from build123d import *

# Parameters (mm, degrees)
SKETCH_1_R      = 60
SKETCH_1_R_2    = 5
EXTRUDE_1_DEPTH = 3
FILLET_1_R      = 2
FILLET_2_R      = 2
FILLET_4_R      = 2


with BuildPart() as part:
    # 草图1 → 凸台-拉伸1 (new body)
    with BuildSketch(Plane.XY):
        Circle(SKETCH_1_R)
        Circle(SKETCH_1_R_2, mode=Mode.SUBTRACT)
        with BuildLine():
            Line((3, 54.918120871), (3, 9.539392014))
            ThreePointArc((3, 9.539392014), (7.071067812, 7.071067812), (9.539392014, 3))
            Line((9.539392014, 3), (54.918120871, 3))
            ThreePointArc((54.918120871, 3), (38.890872965, 38.890872965), (3, 54.918120871))
        make_face(mode=Mode.SUBTRACT)
        with BuildLine():
            Line((-9.539392014, -3), (-54.918120871, -3))
            ThreePointArc((-54.918120871, -3), (-38.890872965, -38.890872965), (-3, -54.918120871))
            Line((-3, -54.918120871), (-3, -9.539392014))
            ThreePointArc((-3, -9.539392014), (-7.071067812, -7.071067812), (-9.539392014, -3))
        make_face(mode=Mode.SUBTRACT)
        with BuildLine():
            Line((9.539392014, -3), (54.918120871, -3))
            ThreePointArc((54.918120871, -3), (38.890872965, -38.890872965), (3, -54.918120871))
            Line((3, -54.918120871), (3, -9.539392014))
            ThreePointArc((3, -9.539392014), (7.071067812, -7.071067812), (9.539392014, -3))
        make_face(mode=Mode.SUBTRACT)
        with BuildLine():
            Line((-3, 9.539392014), (-3, 54.918120871))
            ThreePointArc((-3, 54.918120871), (-38.890872965, 38.890872965), (-54.918120871, 3))
            Line((-54.918120871, 3), (-9.539392014, 3))
            ThreePointArc((-9.539392014, 3), (-7.071067812, 7.071067812), (-3, 9.539392014))
        make_face(mode=Mode.SUBTRACT)
    extrude(amount=EXTRUDE_1_DEPTH)

    # 圆角1
    fillet_1_edges = [part.edges().sort_by_distance(p)[0] for p in [
        (3, 54.918120871, 1.5),
    ]]
    fillet(fillet_1_edges, radius=FILLET_1_R)

    # 圆角2
    fillet_2_edges = [part.edges().sort_by_distance(p)[0] for p in [
        (54.918120871, 3, 1.5),
        (3, -54.918120871, 1.5),
        (54.918120871, -3, 1.5),
        (-54.918120871, -3, 1.5),
        (-3, -54.918120871, 1.5),
        (-3, 54.918120871, 1.5),
        (-54.918120871, 3, 1.5),
    ]]
    fillet(fillet_2_edges, radius=FILLET_2_R)

    # 圆角4
    fillet_4_edges = [part.edges().sort_by_distance(p)[0] for p in [
        (3, 9.539392014, 1.5),
        (9.539392014, 3, 1.5),
        (9.539392014, -3, 1.5),
        (3, -9.539392014, 1.5),
        (-3, -9.539392014, 1.5),
        (-9.539392014, -3, 1.5),
        (-9.539392014, 3, 1.5),
        (-3, 9.539392014, 1.5),
    ]]
    fillet(fillet_4_edges, radius=FILLET_4_R)


solid = part.part
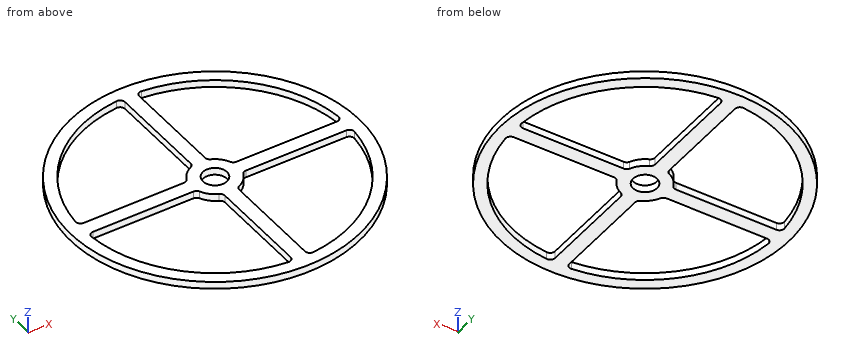
Geometry check sheet. Reference: the model listing, model coordinates, mm. Give positions to 0.01 mm unless a question says otherwise; leave off trailing zeros. Order: outer loops, then holes, each group sorted by start corner. A loop starts at its lowest first (then second) coordinate and runs counter-clockwise, first axis right, second up.
1. Sectioned sample at C-C (z = 1.4). State how many separate pieces and enclosed holes the cut face has, then the cut area to 3 significant figures.
Completed:
separate pieces: 1
enclosed holes: 5
area: 3,140 mm2
2. Sectioned sample at B-B (y = 28). Record the boundary of the cut face in (x, z).
Completed:
outline: (-53.07, 0) - (-47.34, 0) - (-47.34, 3) - (-53.07, 3) - close; (-3, 0) - (3, 0) - (3, 3) - (-3, 3) - close; (47.34, 0) - (53.07, 0) - (53.07, 3) - (47.34, 3) - close
3. Scan lines: line 1 (Y direction, x = 12, z = 2.7); line 2 (Y direction, x = 15.5, z = 1.3); line 3 (X direction, y = -18, z = 1.25). Record each from-to range of solid material in increasing order.
Completed:
line 1: y = -58.79 to -53.67, -3 to 3, 53.67 to 58.79
line 2: y = -57.96 to -52.77, -3 to 3, 52.77 to 57.96
line 3: x = -57.24 to -51.97, -3 to 3, 51.97 to 57.24
4. Sectioned sample at A-A (x = 0). Record the boundary of the cut face in (y, z).
Completed:
outline: (-60, 0) - (-5, 0) - (-5, 3) - (-60, 3) - close; (5, 0) - (60, 0) - (60, 3) - (5, 3) - close
5. Sectioned sample at D-D (x = -20.5). Record the boundary of the cut face in (y, z).
Completed:
outline: (-56.39, 0) - (-51.04, 0) - (-51.04, 3) - (-56.39, 3) - close; (-3, 0) - (3, 0) - (3, 3) - (-3, 3) - close; (51.04, 0) - (56.39, 0) - (56.39, 3) - (51.04, 3) - close
6. Depth check by flat-ended pin: pin 1 (1.5 mm diameter, centred on x = -35, z = 1.5, fed in from -Y); pin 2 (1 mm diameter, centred on y = 4, z = 2.5, fed in from -X); pin 3 (0.9 mm diameter, centred on y = -26.5, z = 1.5, fed in from +X); pin 4 (10 mm diameter, centred on x = 46.5, y = -18, fed in from -Z). Enter the tip coordinate at first touch or a pass-through.
Completed:
pin 1: stops at y = -49.26
pin 2: stops at x = -59.9
pin 3: stops at x = 54.05
pin 4: passes through
